from build123d import *

# Parameters (mm, degrees)
SKETCH2_W           = 279.4
SKETCH2_H           = 279.4
BOSS_EXTRUDE2_DEPTH = 304.8
SHELL2_T            = -3.175
SKETCH4_W           = 76.2
SKETCH4_H           = 25.4
CUT_EXTRUDE2_DEPTH  = 280.4
BOSS_EXTRUDE5_DEPTH = 3.175
SKETCH6_R           = 12.7
CUT_EXTRUDE3_DEPTH  = 305.8


with BuildPart() as part:
    # Sketch2 → Boss-Extrude2 (new body)
    with BuildSketch(Plane.XY):
        with Locations((139.7, 139.7)):
            Rectangle(SKETCH2_W, SKETCH2_H)
    extrude(amount=BOSS_EXTRUDE2_DEPTH)

    # Shell2
    shell2_openings = [part.faces().sort_by_distance(p)[0] for p in [
        (139.7, 139.7, 304.8),
    ]]
    offset(amount=SHELL2_T, openings=shell2_openings, kind=Kind.INTERSECTION)

    # Sketch4 → Cut-Extrude2 (cut, through all)
    with BuildSketch(Plane.ZY):
        with Locations((266.7, 139.7)):
            Rectangle(SKETCH4_W, SKETCH4_H)
    extrude(amount=-CUT_EXTRUDE2_DEPTH, mode=Mode.SUBTRACT)

    # Sketch5 → Boss-Extrude5 (add)
    with BuildSketch(Plane(origin=(279.4, 0, 0), x_dir=(0, 0, -1), z_dir=(1, 0, 0))):
        Polygon((0, 63.5), (0, 0), (38.1, 0), (38.1, 19.05), (30.767651581, 19.05), (23.435303163, 31.75), (30.767651581, 44.45), (38.1, 44.45), (38.1, 63.5), align=None)
        with BuildLine():
            Line((38.1, 19.05), (38.1, 0))
            ThreePointArc((38.1, 0), (69.85, 31.75), (38.1, 63.5))
            Line((38.1, 63.5), (38.1, 44.45))
            Line((38.1, 44.45), (45.432348419, 44.45))
            Line((45.432348419, 44.45), (52.764696837, 31.75))
            Line((52.764696837, 31.75), (45.432348419, 19.05))
            Line((45.432348419, 19.05), (38.1, 19.05))
        make_face()
    boss_extrude5 = extrude(amount=-BOSS_EXTRUDE5_DEPTH)

    # Mirror1: Boss-Extrude5 across plane
    add(boss_extrude5.mirror(Plane(origin=(139.7, 0, 0), x_dir=(0, 0, 1), z_dir=(1, 0, 0))))

    # Sketch6 → Cut-Extrude3 (cut, through all)
    with BuildSketch(Plane(origin=(0, 0, 0), x_dir=(-1, 0, 0), z_dir=(0, 0, -1))):
        with Locations((-139.7, 139.7)):
            Circle(SKETCH6_R)
    extrude(amount=-CUT_EXTRUDE3_DEPTH, mode=Mode.SUBTRACT)


solid = part.part
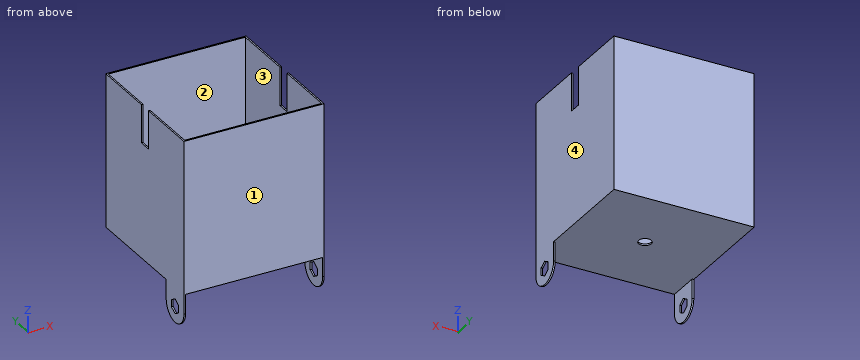
Could you check a few things on this model? Use its own coordinates, in mm. Face numbers are marked on the shaded views. Coordinates: 2 decimals unless noted, no trailing zeros. Loops run counter-clockwise (first coordinate to the right, second up) from the corner with the lowest first, then second, coordinate; pieces in that order, holes last.
1. Imagine slicing it at C-C (x = 139.7). Please give me the cut outline in (y, z) (3 decimals).
2. Imagine slicing it at B-B (y = 139.7). Please give me the cut outline in (x, z) (3 decimals).
3. Imagine slicing it at D-D (z = 209). Please give me the cut outline in (x, y) (3 decimals), and give its area (3 significant figures).
4. We'd pull the mould along Y, two halves only. Please class the marked faces 1, 2, 3 and 4: released by +Y, released by -Y, zero draft, split by the parting line, or undercut.
5. For P1, Ø1.6, axis at x = 2, y = 137.5, coming from the +Z side; P2, Ø1.5, axis at x = 234.5, y = 173.5, coming from the -Z side; P3, Ø1.6, axis at x = 278, z = -11.5, coming from the +Y side; P4, Ø15, axis at x = 139.7, y = 139.7, coming from the +Z side, each with a flat end and sliding along its axis, tell me the tip position at first contact or that it passes through.
6. I need wall thicknesses on L1, parallel to X at y = 195, z = 83 (3 decimals); L2, parallel to Y at x = 139, z = 1. Which ranges of each line are inside material? Lowest first, please.
7. Imagine slicing it at A-A (z = -12.5). Please give me the cut outline in (x, y) (3 decimals).
Computed values:
1. outline: (0, 0) - (127, 0) - (127, 3.175) - (3.175, 3.175) - (3.175, 304.8) - (0, 304.8) - close; (152.4, 0) - (279.4, 0) - (279.4, 304.8) - (276.225, 304.8) - (276.225, 3.175) - (152.4, 3.175) - close
2. outline: (0, 0) - (127, 0) - (127, 3.175) - (3.175, 3.175) - (3.175, 228.6) - (0, 228.6) - close; (152.4, 0) - (279.4, 0) - (279.4, 228.6) - (276.225, 228.6) - (276.225, 3.175) - (152.4, 3.175) - close
3. outline: (0, 0) - (279.4, 0) - (279.4, 279.4) - (0, 279.4) - close; hole (3.175, 3.175) - (276.225, 3.175) - (276.225, 276.225) - (3.175, 276.225) - close
3. area: 3,510 mm2
4. face 1: released by -Y
4. face 2: undercut
4. face 3: undercut
4. face 4: zero draft
5. P1: stops at z = 228.6
5. P2: stops at z = 0
5. P3: stops at y = 63.5
5. P4: passes through
6. L1: x = 0 to 3.175, 276.225 to 279.4
6. L2: y = 0 to 127.02, 152.38 to 279.4
7. outline: (0, 0) - (3.175, 0) - (3.175, 63.5) - (0, 63.5) - close; (276.225, 0) - (279.4, 0) - (279.4, 63.5) - (276.225, 63.5) - close
